Input: part model. Units: mm. Frame: model coordinates. Face numbers are marked on the shaded views. Give positions to 0.01 mm unless a question says otherwise; leave off trailing zeros. Order: outer loops, then holes, each group sorted by start corner. A loop starts at its lowest first (then second) coordinate and runs counter-clockwise, first axis right, second up. Notation, with made-up numbers: (87, -24.5) - (137, -24.5) arc R18 cw to (137, 2.5) - close; hole circle Ø5 at (57, 15.5). An arc over 180 degrees is marked (long way). Use a Markdown table: item, result.
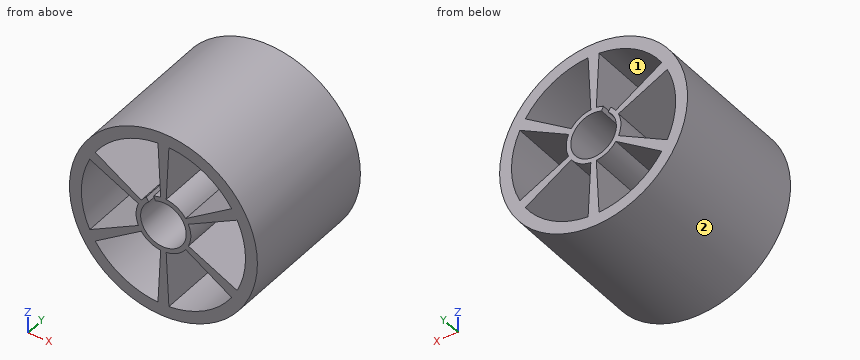
from build123d import *

# Parameters (mm, degrees)
F0_R     = 25.75
F1_DEPTH = 41


with BuildPart() as f1:
    # F0 (on Front) → F1 (new body)
    with BuildSketch(Plane.XZ):
        Circle(F0_R)
        with BuildLine():
            ThreePointArc((-1.5, -22.449944), (-11.250362, -19.485363), (-18.692687, -12.523316))
            Line((-18.692687, -12.523316), (-6.088184, -4.379957))
            ThreePointArc((-6.088184, -4.379957), (-3.75, -6.495191), (-0.749062, -7.4625))
            Line((-0.749062, -7.4625), (-1.5, -22.449944))
        make_face(mode=Mode.SUBTRACT)
        with BuildLine():
            ThreePointArc((18.692222, -12.52401), (11.249638, -19.48578), (1.499166, -22.45))
            Line((1.499166, -22.45), (0.749062, -7.4625))
            ThreePointArc((0.749062, -7.4625), (3.75, -6.495191), (6.088184, -4.379957))
            Line((6.088184, -4.379957), (18.692222, -12.52401))
        make_face(mode=Mode.SUBTRACT)
        with BuildLine():
            ThreePointArc((20.192222, 9.925934), (22.5, -0.000418), (20.191854, -9.926684))
            Line((20.191854, -9.926684), (6.837246, -3.082543))
            ThreePointArc((6.837246, -3.082543), (7.5, 0), (6.837246, 3.082543))
            Line((6.837246, 3.082543), (20.192222, 9.925934))
        make_face(mode=Mode.SUBTRACT)
        with BuildLine():
            ThreePointArc((-20.192222, -9.925934), (-22.5, 0.000418), (-20.191854, 9.926684))
            Line((-20.191854, 9.926684), (-6.837246, 3.082543))
            ThreePointArc((-6.837246, 3.082543), (-7.5, 0), (-6.837246, -3.082543))
            Line((-6.837246, -3.082543), (-20.192222, -9.925934))
        make_face(mode=Mode.SUBTRACT)
        with BuildLine():
            ThreePointArc((-2.186485, 5.855065), (3.143303, -5.40205), (-4.009937, 4.794049))
            Line((-4.009937, 4.794049), (-4.714155, 5.833245))
            ThreePointArc((-4.714155, 5.833245), (-5.44983, 5.152607), (-6.088184, 4.379957))
            Line((-6.088184, 4.379957), (-18.692222, 12.52401))
            ThreePointArc((-18.692222, 12.52401), (-11.249638, 19.48578), (-1.499166, 22.45))
            Line((-1.499166, 22.45), (-0.749062, 7.4625))
            ThreePointArc((-0.749062, 7.4625), (-1.737374, 7.295994), (-2.69466, 6.9992))
            Line((-2.69466, 6.9992), (-2.186485, 5.855065))
        make_face(mode=Mode.SUBTRACT)
        with BuildLine():
            Line((0.749062, 7.4625), (1.5, 22.449944))
            ThreePointArc((1.5, 22.449944), (11.250362, 19.485363), (18.692687, 12.523316))
            Line((18.692687, 12.523316), (6.088184, 4.379957))
            ThreePointArc((6.088184, 4.379957), (3.75, 6.495191), (0.749062, 7.4625))
        make_face(mode=Mode.SUBTRACT)
    extrude(amount=F1_DEPTH)


solid = f1.part
1. Material intervals for line 1 along Z through (x, y) = (0, -13); line 2 along X through (y, z) = (-5.5, -1.5); line 3 along X through (y, z) = (-6, 3.5), sorted ascending.
Response:
| item | result |
|---|---|
| line 1 | z = -25.75 to -6.25, 6.25 to 25.75 |
| line 2 | x = -25.71 to -22.45, -7.35 to -6.07, 6.07 to 7.35, 22.45 to 25.71 |
| line 3 | x = -25.51 to -22.23, -7.65 to -5.18, 5.18 to 7.65, 22.23 to 25.51 |
2. Mould query, pull axis X, two halves, no side actions, for the marked faces 1 and 2. Classes: pulls with the +X half, pulls with the -X half, needs draft (parallel to the pull), parting line crosses it, or undercut.
Response:
| item | result |
|---|---|
| face 1 | undercut |
| face 2 | parting line crosses it |
3. Section query D-D (x = -9). Return loops of the section in (y, z).
Response:
| item | result |
|---|---|
| outline | (-41, -24.13) - (0, -24.13) - (0, -20.62) - (-41, -20.62) - close; (-41, -6.26) - (0, -6.26) - (0, -4.19) - (-41, -4.19) - close; (-41, 4.19) - (0, 4.19) - (0, 6.26) - (-41, 6.26) - close; (-41, 20.62) - (0, 20.62) - (0, 24.13) - (-41, 24.13) - close |
4. Section query B-B (z = 0). Return loops of the section in (x, y).
Response:
| item | result |
|---|---|
| outline | (-25.75, -41) - (-22.5, -41) - (-22.5, 0) - (-25.75, 0) - close; (-7.5, -41) - (-6.25, -41) - (-6.25, 0) - (-7.5, 0) - close; (6.25, -41) - (7.5, -41) - (7.5, 0) - (6.25, 0) - close; (22.5, -41) - (25.75, -41) - (25.75, 0) - (22.5, 0) - close |
5. Section query C-C (x = 0). Return loops of the section in (y, z), then the cut area to 3 significant figures.
Response:
| item | result |
|---|---|
| outline | (-41, -25.75) - (0, -25.75) - (0, -6.25) - (-41, -6.25) - close; (-41, 6.25) - (0, 6.25) - (0, 25.75) - (-41, 25.75) - close |
| area | 1,600 mm^2 |
6. Section query A-A (y = -10). State how many separate pieces and enclosed holes the cut face has, then the cut area to 3 significant figures.
Response:
| item | result |
|---|---|
| separate pieces | 1 |
| enclosed holes | 6 |
| area | 746 mm^2 |
7. Pin query (flat end, axial travel): pin 1 (4 mm diameter, centred on y = -6.5, z = -17, fed in from -X); pin 2 (4 mm diameter, centred on y = -35.5, z = -14, fed in from -X); pin 3 (1.5 mm diameter, centred on y = -22.5, z = -1.5, fed in from -X). Return the tip coordinate at first contact, or that it passes through.
Response:
| item | result |
|---|---|
| pin 1 | stops at x = -20.93 |
| pin 2 | stops at x = -22.78 |
| pin 3 | stops at x = -25.74 |
